from build123d import *

# Parameters (mm, degrees)
F0_R     = 7
F1_DEPTH = 2
F2_SIZE  = 1
F3_R     = 5
F4_DEPTH = 6
F5_SIZE  = 0.25
F7_D     = 6
F7_DEPTH = 4
F7_TIP   = 1.8025818571


with BuildPart() as f1:
    # F0 (on Top) → F1 (new body)
    with BuildSketch(Plane.XY):
        Circle(F0_R)
    extrude(amount=F1_DEPTH)

    # F2
    f2_edges = [f1.edges().sort_by_distance(p)[0] for p in [
        (-7, 0, 2),
    ]]
    chamfer(f2_edges, length=F2_SIZE)

    # F3 (on face) → F4 (join)
    with BuildSketch(Plane(origin=(0, 0, 0), x_dir=(1, 0, 0), z_dir=(0, 0, -1))):
        Circle(F3_R)
    extrude(amount=F4_DEPTH)

    # F5
    f5_edges = [f1.edges().sort_by_distance(p)[0] for p in [
        (-5, 0, -6),
    ]]
    chamfer(f5_edges, length=F5_SIZE)

    # F7
    with Locations(Plane(origin=(0, 0, -6), x_dir=(1, 0, 0), z_dir=(0, 0, -1))):
        with Locations((0, 0)):
            Hole(F7_D / 2, depth=F7_DEPTH)
            with Locations((0, 0, -(F7_DEPTH + F7_TIP / 2))):  # 118° drill point
                Cone(0, F7_D / 2, F7_TIP, mode=Mode.SUBTRACT)


solid = f1.part
Here's how the part is built. I have some questions about the finished solid (model axes, mm). A direction names the side the tool comes from. Give positions to 0.01 mm unless a question says otherwise; leave off trailing zeros. Order: outer loops, then holes, each group sorted by start corner. A loop starts at its lowest first (then second) coordinate and runs counter-clockwise, first axis right, second up. Notation, with made-up numbers: M 17.5,40 L 72.5,40 A15 ccw 72.5,55 Z; hole C 45.25,83 d7. An arc over 180 degrees is marked long. Answer as a JSON object with one key per item and string values. Group by question number.
1) I'm going to push flat-ended pins straight in: pin 1 Ø2 at (x, y) = (-1, -5.5) entering from -Z; pin 2 Ø1 at (x, z) = (-1, -4) entering from -Y. Where does each tip first touch, or does it pass through?
2) Suppose I cut it at B-B, the plane z = -1.25. Write out the boundary of the cut face in (x, y), plus the area to 3 significant figures.
3) On a 3-axis mill with a long thin cutter (end or side, diameter ignored), from which of +Z, -Z, +X, -X, +Y, -Y can I reach the whole of each face in a straight line? I mean faces 1 (the cylindrical face through (3, 0, -4)), 2 (the flat face through (3, 1, -6)). Say none if no direction works.
4) Suppose I cut it at A-A, the plane z = -5.5. Write out the boundary of the cut face in (x, y).
5) Please list where these lines run through material, in increasing order: L1, parallel to Y at x = 0, z = -4.8; L2, parallel to Z at x = -4.75, y = -1.75; L3, parallel to Y at x = -4, z = -4. Write a range as [from, to].
Results found:
{
 "1": {"pin 1": "z = -6", "pin 2": "y = -4.97"},
 "2": {"outline": "C 0,0 d10; hole C 0,0 d3.5", "area": "68.9 mm²"},
 "3": {"face 1": "-Z", "face 2": "-Z, +X, -X, +Y, -Y"},
 "4": {"outline": "C 0,0 d10; hole C 0,0 d6"},
 "5": {"L1": "[-5, -3], [3, 5]", "L2": "[0, 2]", "L3": "[-3, 3]"}
}
